CAD build for the part. Positions are in the model's coordinates, mm. A direction names the side the tool comes from. Give positions to 0.01 mm unless a question says otherwise; leave off trailing zeros. Loops run counter-clockwise (first coordinate to the right, second up) from the corner with the lowest first, then second, coordinate; pieces in that order, holes last. Notation, with made-up numbers: M 53,-29.75 L 83,-29.75 A18 ccw 83,-14.75 Z; hole C 69.5,17.25 d4. An arc over 180 degrees is marked long. One line per question, with ' | ' between items.
```python
from build123d import *

# Parameters (mm, degrees)
SKETCH1_R               = 35
SKETCH1_R_2             = 22.5
BOSS_EXTRUDE1_DEPTH     = 18
CUT_EXTRUDE1_DEPTH      = 53.668776329
CUT_EXTRUDE1_DEPTH_BACK = 53.668776329
SKETCH2_R               = 5
SKETCH2_W               = 35
SKETCH2_H               = 10
BOSS_EXTRUDE2_START     = 18
SKETCH3_R               = 5
BOSS_EXTRUDE2_DEPTH     = 13
MIRROR2_START           = 18
MIRROR2_COPY_1_SKETCH_R = 5
MIRROR2_COPY_1_DEPTH    = 13
BOSS_EXTRUDE4_START     = -10
BOSS_EXTRUDE4_OUTLINE_R = 7.5
BOSS_EXTRUDE4_DEPTH     = 20


# Read off the part's stored shape, not the designer's step: Boss-Extrude4
with BuildPart() as part:
    # Sketch1 → Boss-Extrude1 (new, symmetric)
    with BuildSketch(Plane(origin=(0, 0, 0), x_dir=(1, 0, 0), z_dir=(0, 1, 0))):
        with Locations(Location((0, 0, 0), (0, 0, 270))):
            Circle(SKETCH1_R)
        with Locations(Location((0, 0, 0), (0, 0, 270))):
            Circle(SKETCH1_R_2, mode=Mode.SUBTRACT)
    extrude(amount=BOSS_EXTRUDE1_DEPTH, both=True)

    # Sketch2 → Cut-Extrude1 (cut, two sides: drawn at the far end of the back side and taken through both)
    with BuildSketch(Plane.XY.offset(-CUT_EXTRUDE1_DEPTH_BACK)):
        Circle(SKETCH2_R)
        with Locations((17.5, 0)):
            Rectangle(SKETCH2_W, SKETCH2_H)
    extrude(amount=CUT_EXTRUDE1_DEPTH + CUT_EXTRUDE1_DEPTH_BACK, mode=Mode.SUBTRACT)

    # Sketch3 → Boss-Extrude2 (add)
    with BuildSketch(Plane(origin=(0, 0, 0), x_dir=(1, 0, 0), z_dir=(0, 1, 0)).offset(BOSS_EXTRUDE2_START)):
        with BuildLine():
            Line((28.284271247, -42.426406871), (16.646014639, -30.788150263))
            ThreePointArc((16.646014639, -30.788150263), (24.748737342, -24.748737342), (30.788150263, -16.646014639))
            Line((30.788150263, -16.646014639), (42.426406871, -28.284271247))
            ThreePointArc((42.426406871, -28.284271247), (42.426406871, -42.426406871), (28.284271247, -42.426406871))
        make_face()
        with Locations(Location((35.355339059, -35.355339059, 0), (0, 0, 90))):
            Circle(SKETCH3_R, mode=Mode.SUBTRACT)
    boss_extrude2 = extrude(amount=-BOSS_EXTRUDE2_DEPTH)

    # Mirror1: Boss-Extrude2 across plane
    add(boss_extrude2.mirror(Plane.XY))

    # Mirror2: Boss-Extrude2 across plane
    add(boss_extrude2.mirror(Plane.ZX))

    # Mirror2 copy 1 sketch → Mirror2 copy 1 (add)
    with BuildSketch(Plane.XZ.offset(MIRROR2_START)):
        with BuildLine():
            Line((28.284271247, -42.426406871), (16.646014639, -30.788150263))
            ThreePointArc((16.646014639, -30.788150263), (24.748737342, -24.748737342), (30.788150263, -16.646014639))
            Line((30.788150263, -16.646014639), (42.426406871, -28.284271247))
            ThreePointArc((42.426406871, -28.284271247), (42.426406871, -42.426406871), (28.284271247, -42.426406871))
        make_face()
        with Locations(Location((35.355339059, -35.355339059, 0), (0, 0, 90))):
            Circle(MIRROR2_COPY_1_SKETCH_R, mode=Mode.SUBTRACT)
    extrude(amount=-MIRROR2_COPY_1_DEPTH)

    # Boss-Extrude4 outline → Boss-Extrude4 (add)
    with BuildSketch(Plane.XY.offset(BOSS_EXTRUDE4_START)):
        with BuildLine():
            Line((-22.5, 18), (-60, 18))
            ThreePointArc((-60, 18), (-78, 0), (-60, -18))
            Line((-60, -18), (-22.5, -18))
            Line((-22.5, -18), (-22.5, 18))
        make_face()
        with Locations((-60, 0)):
            Circle(BOSS_EXTRUDE4_OUTLINE_R, mode=Mode.SUBTRACT)
    extrude(amount=BOSS_EXTRUDE4_DEPTH)


solid = part.part
```
Item 1: Mould opens along X. For faces 4 (the flat face through (17, -18, 20)), 5 (the cylindrical face through (-67.493, 0.33, -0.14)), 6 (the flat face through (36.526, -11.591, -22.384)) say: pulls with the +X half, pulls with the -X half, needs draft (parallel to the pull), parting line crosses it, or undercut.
Conclusion:
face 4: needs draft | face 5: undercut | face 6: pulls with the +X half
Item 2: Drop flat-ended pins along their axis: P1, Ø8, axis at y = -4.5, z = -5, coming from the +X side; P2, Ø17, axis at x = -60, y = 0, coming from the +Z side; P3, Ø8, axis at x = 35.36, z = -35.36, coming from the +Y side; P4, Ø8, axis at x = -51.5, y = 13, coming from the -Z side. Give the stop position or say it passes through.
Conclusion:
P1: x = 34.98 | P2: z = 10 | P3: through | P4: z = -10
Item 3: Drill centre lines: line 1 along Y through (x, z) = (13.5, 32); line 2 along Z through (x, y) = (-44.5, -0.5); line 3 along X through (y, z) = (-1.5, 8). Where is each one in solid material? Low to high. Write a range as [from, to].
Conclusion:
line 1: [-18, -5], [5, 18] | line 2: [-10, 10] | line 3: [-77.94, -67.35], [-52.65, -21.03]
Item 4: Saw through at C-C on y = 0. Give the cut face in (x, z).
Conclusion:
outline: M -78,-10 L -67.5,-10 L -67.5,10 L -78,10 Z; M -52.5,-10 L -33.54,-10 A35 ccw -5,-34.64 L -5,-21.94 A22.5 cw -5,21.94 L -5,34.64 A35 ccw -33.54,10 L -52.5,10 Z
Item 5: Saw through at A-A on z = 0. Give the cut face in (x, y), and give its area (3 significant figures).
Conclusion:
outline: M -60,-18 L -22.5,-18 L -22.5,18 L -60,18 A18 ccw Z; M 22.5,-18 L 35,-18 L 35,-5 L 22.5,-5 Z; M 22.5,5 L 35,5 L 35,18 L 22.5,18 Z; hole C -60,0 d15 | area: 2,010 mm²
Item 6: Saw through at B-B on y = -13.5. Give the cut face in (x, z).
Conclusion:
outline: M -71.91,-10 L -33.54,-10 A35 ccw 16.65,-30.79 L 28.28,-42.43 A10 ccw 42.43,-28.28 L 30.79,-16.65 A35 ccw 30.79,16.65 L 42.43,28.28 A10 ccw 28.28,42.43 L 16.65,30.79 A35 ccw -33.54,10 L -71.91,10 Z; hole C 0,0 d45; hole C 35.36,-35.36 d10; hole C 35.36,35.36 d10
Item 7: Saw through at D-D on x = -11. Give the cut face in (y, z).
Conclusion:
outline: M -18,-33.23 L 18,-33.23 L 18,-19.63 L -18,-19.63 Z; M -18,19.63 L 18,19.63 L 18,33.23 L -18,33.23 Z
Item 8: 3-axis set-ups, long thin cutter, end or side, ignore diameter. For faces 1 (the flat face through (27, -5, -1)), 2 (the flat face through (-51, 0, 10)), 3 (the flat face through (36.526, 11.591, -22.384)): which of +Z, -Z, +X, -X, +Y, -Y reach the whole face in a straight line?
Conclusion:
face 1: +Z, -Z, +X | face 2: +Z, -X, +Y, -Y | face 3: +X, +Y, -Y
